```python
from build123d import *

# Parameters (mm, degrees)
BOSS_EXTRUDE1_DEPTH = 75
SKETCH2_W           = 8.8
SKETCH2_H           = 20
CUT_EXTRUDE1_DEPTH  = 0.7


with BuildPart() as part:
    # Sketch1 → Boss-Extrude1 (new body, symmetric)
    with BuildSketch(Plane.XY):
        Polygon((4.75, 4.75), (4.75, -4.75), (-4.75, -4.75), (-4.75, -4.05), (4.05, -4.05), (4.05, 4.05), (-4.75, 4.05), (-4.75, 4.75), align=None)
    extrude(amount=BOSS_EXTRUDE1_DEPTH, both=True)

    # Sketch2 → Cut-Extrude1 (cut)
    with BuildSketch(Plane(origin=(0, 4.75, 0), x_dir=(1, 0, 0), z_dir=(0, 1, 0))):
        with Locations((-0.35, 65)):
            Rectangle(SKETCH2_W, SKETCH2_H)
    cut_extrude1 = extrude(amount=-CUT_EXTRUDE1_DEPTH, mode=Mode.SUBTRACT)

    # Mirror1: Cut-Extrude1 across plane
    add(cut_extrude1.mirror(Plane.XY), mode=Mode.SUBTRACT)


solid = part.part
```
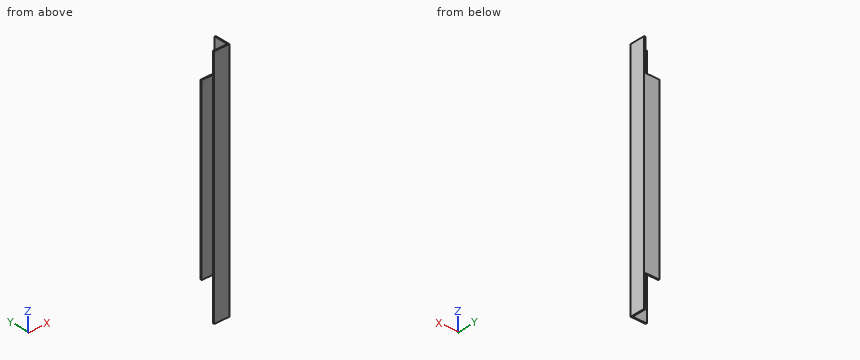
Geometry check sheet. Reference: the model listing, model coordinates, mm. Give positions to 0.01 mm unless a question says otherwise; leave off trailing zeros. Order: outer loops, then holes, each group sorted by start corner. A loop starts at its lowest first (then second) coordinate and runs counter-clockwise, first axis right, second up. Notation, with made-up numbers: (0, -5) - (21, -5) arc R28 cw to (21, 25) - close; hole circle Ø9 at (75, 89.5). An arc over 180 degrees is marked (long way). Answer in a Markdown table with one row per item. Add a question column.
Q1. Cross-section at C-C, the plane y = 1. Enter the section's corners in (x, z), then the cut area to 3 significant figures.
Q2. Cross-section at A-A, the plane x = 2.75. Enter the section's corners in (y, z), then the cut area to 3 significant figures.
Q3. Material ranges on probe 1 along Y at (x, z) = (0.25, 41.5); probe 2 along X at (y, z) = (3, -22.5), recorded low to high. Write a range as from..to.
Q4. Gauge pin test, flat ends, axial feed: pin 1 (1.5 mm diameter, centred on x = -3, y = -2, fed in from +Z); pin 2 (5 mm diameter, centred on y = -0.5, z = -14.5, fed in from -X). Record the tip position at first contact, or that the pin passes through.
Q5. Cross-section at B-B, the plane z = 36.5. Enter the section's corners in (x, y), then the cut area to 3 significant figures.
Check values:
| question | item | result |
|---|---|---|
| 1 | outline | (4.05, -75) - (4.75, -75) - (4.75, 75) - (4.05, 75) - close |
| 1 | area | 105 mm^2 |
| 2 | outline | (-4.75, -75) - (-4.05, -75) - (-4.05, 75) - (-4.75, 75) - close; (4.05, -55) - (4.75, -55) - (4.75, 55) - (4.05, 55) - close |
| 2 | area | 182 mm^2 |
| 3 | probe 1 | y = -4.75..-4.05, 4.05..4.75 |
| 3 | probe 2 | x = 4.05..4.75 |
| 4 | pin 1 | passes through |
| 4 | pin 2 | stops at x = 4.05 |
| 5 | outline | (-4.75, -4.75) - (4.75, -4.75) - (4.75, 4.75) - (-4.75, 4.75) - (-4.75, 4.05) - (4.05, 4.05) - (4.05, -4.05) - (-4.75, -4.05) - close |
| 5 | area | 19.0 mm^2 |
